Read the model definition and answer for the solid it produces. Units are mm, in the model's axes. A direction names the side the tool comes from. Coordinates: 2 decimals unless noted, no trailing zeros. Loops run counter-clockwise (first coordinate to the right, second up) from the corner with the lowest first, then second, coordinate; pieces in that order, holes last. Notation, with made-up numbers: (8.5, 20.5) -> (38.5, 20.5) arc R17 ccw to (38.5, 51.5) -> close; hole circle Ø2 at (57, 7.25). An arc over 180 degrees is marked (long way). Answer as a JSON object with one key per item and string values. Group by question number.
1) Flat-ended cylindrical pins translate along their axes: P1, Ø4, axis at x = -25.4, y = -63.5, coming from the +Z side; P2, Ø1.4, axis at x = -25, y = -64.5, coming from the -Z side; P3, Ø3, axis at x = 31.75, y = -63.5, coming from the +Z side; P4, Ø5, axis at x = -12.5, y = -17, coming from the +Z side. Find the tip coordinate at first contact, or state that the pin passes through.
2) Which of the six approach directions +Z, -Z, +X, -X, +Y, -Y give full straight-line access (tool end or side, diameter ignored) to faces 4 (the face through (-31.853, -61.153, -6.367)), 5 (the face through (25.297, -65.847, -25.383)), 6 (the face through (-32, -38, 0))?
3) Section C-C, the plane z = -13.5 is taken. Give the vertices of the cut face in (x, y).
4) Consider probe 1 along Y at (x, z) = (-25.4, -28.55); probe 2 along X at (y, z) = (-12.7, -28.05); probe 3 along Y at (x, z) = (31.75, -6.55). Determine where each line is inside the solid, lowest interval first. Write a range as [from, to].
5) Section A-A, the plane z = -1.5 is taken. Give the vertices of the cut face in (x, y), plus the area to 3 significant figures.
6) Section B-B, the plane x = -31.75 is taken. Give the vertices of the cut face in (y, z), plus the area to 3 significant figures.
7) Section D-D, the plane y = -30.5 is taken. Give the vertices of the cut face in (x, z).
8) Determine the mould class of faces 1 (the face through (-23.316, -11.616, -25.383)), 2 (the face through (26.3, -10.53, -25.38)), 3 (the face through (38.1, -38, -16)) for opening direction Y: released by +Y, released by -Y, zero draft, split by the parting line, or undercut.
Autodesk Inventor part; units mm, degrees
ref_plane "YZ Plane" through (0, 0, 0) normal (1, 0, 0) x (0, 1, 0)
ref_plane "XZ Plane" through (0, 0, 0) normal (0, 1, 0) x (-1, 0, 0)
ref_plane "XY Plane" through (0, 0, 0) normal (0, 0, 1) x (1, 0, 0)
sketch "Sketch18" plane through (0, 0, 0) normal (0, 1, 0) x (-1, 0, 0)
  arc A0 (-25.4, 0) -> (25.4, 0) centre (0, 0) ccw
  line L0 (-38.1, 0) -> (-38.1, -31.75)
  line L1 (-38.1, -31.75) -> (38.1, -31.75)
  line L2 (38.1, -31.75) -> (38.1, 0)
  line L3 (38.1, 31.75) -> (-38.1, -31.75) construction
  line L4 (-38.1, 31.75) -> (38.1, -31.75) construction
  line L5 (38.1, 0) -> (25.4, 0)
  line L6 (-25.4, 0) -> (-38.1, 0)
  dimension "d78" = 50.8
  dimension "d79" = 6.35
  dimension "d80" = 12.7
extrude "Extrusion9" add sketch "Sketch18" against normal blind 76.2
sketch "Sketch19" plane through (-38.1, 0, 0) normal (0, 0, 1) x (1, 0, 0)
  line L0 (0, 0) -> (0, -76.2)
  line L1 (12.7, 0) -> (12.7, -76.2)
  line L2 (63.5, 0) -> (63.5, -76.2)
  line L3 (76.2, 0) -> (76.2, -76.2)
  line L4 (76.2, -76.2) -> (63.5, -76.2)
  line L5 (12.7, -76.2) -> (0, -76.2)
  line L6 (0, 0) -> (12.7, 0)
  line L7 (63.5, 0) -> (76.2, 0)
  line L8 (6.35, -63.5) -> (69.85, -63.5) construction
  line L9 (69.85, -63.5) -> (69.85, -12.7) construction
  line L10 (69.85, -12.7) -> (6.35, -12.7) construction
  line L11 (6.35, -12.7) -> (6.35, -63.5) construction
  line L12 (63.5, -76.2) -> (12.7, -76.2) construction
  line L13 (12.7, 0) -> (63.5, 0) construction
  point P0 (38.1, 0)
  dimension "d83" = 6.35
  dimension "d84" = 6.35
  dimension "d85" = 12.7
  dimension "d86" = 12.7
hole "Hole3" at (-31.75, -12.7, 0) at (31.75, -12.7, 0) at (31.75, -63.5, 0) at (-31.75, -63.5, 0) direction (0, 0, -1) diameter 4.699 depth 7.1501 counterbore diameter 4.8514 counterbore depth 5.5626
sketch "Sketch20" plane through (38.1, 0, -31.75) normal (0, 0, -1) x (-1, 0, 0)
  line L0 (76.2, 0) -> (76.2, -76.2)
  line L1 (0, 0) -> (76.2, 0)
  line L2 (0, 0) -> (0, -76.2)
  line L3 (76.2, -76.2) -> (0, -76.2)
  line L4 (12.7, -63.5) -> (63.5, -63.5) construction
  line L5 (63.5, -63.5) -> (63.5, -12.7) construction
  line L6 (63.5, -12.7) -> (12.7, -12.7) construction
  line L7 (12.7, -12.7) -> (12.7, -63.5) construction
  line L8 (12.7, -63.5) -> (63.5, -12.7) construction
  line L9 (63.5, -63.5) -> (12.7, -12.7) construction
  line L10 (0, 0) -> (0, -76.2) construction
  point P0 (38.1, 0)
  point P1 (38.1, -38.1)
  dimension "d94" = 12.7
  dimension "d95" = 12.7
  dimension "d96" = 12.7
  dimension "d97" = 12.7
hole "Hole4" at (25.4, -12.7, -31.75) at (-25.4, -12.7, -31.75) at (-25.4, -63.5, -31.75) at (25.4, -63.5, -31.75) direction (0, 0, 1) diameter 4.699 depth 7.1501 counterbore diameter 4.8514 counterbore depth 5.5626
equation "\"d78\" = legDiameter"
equation "\"d81\" = legPartHeight"
equation "\"legDiameter\" = 50.8"
equation "\"legWalThickness\" = 3.175"
equation "\"legPartHeight\" = 76.2"
properties part number "clampForMeadeTripodLeg"
Determined:
{
 "1": {"P1": "z = 0", "P2": "z = -24.6", "P3": "z = -7.15", "P4": "z = -20.5"},
 "2": {"face 4": "+Z", "face 5": "-Z", "face 6": "+Z, +X, -X, +Y, -Y"},
 "3": {"outline": "(-38.1, -76.2) -> (-21.52, -76.2) -> (-21.52, 0) -> (-38.1, 0) -> close; (21.52, -76.2) -> (38.1, -76.2) -> (38.1, 0) -> (21.52, 0) -> close"},
 "4": {"probe 1": "[-76.2, -65.93], [-61.07, -15.13], [-10.27, 0]", "probe 2": "[-38.1, -27.83], [-22.97, 22.97], [27.83, 38.1]", "probe 3": "[-76.2, -65.85], [-61.15, -15.05], [-10.35, 0]"},
 "5": {"outline": "(-38.1, -76.2) -> (-25.36, -76.2) -> (-25.36, 0) -> (-38.1, 0) -> close; (25.36, -76.2) -> (38.1, -76.2) -> (38.1, 0) -> (25.36, 0) -> close; hole circle Ø4.85 at (-31.75, -63.5); hole circle Ø4.85 at (-31.75, -12.7); hole circle Ø4.85 at (31.75, -63.5); hole circle Ø4.85 at (31.75, -12.7)", "area": "1,870 mm²"},
 "6": {"outline": "(-76.2, -31.75) -> (0, -31.75) -> (0, 0) -> (-10.27, 0) -> (-10.27, -5.56) -> (-10.35, -5.56) -> (-10.35, -7.15) -> (-15.05, -7.15) -> (-15.05, -5.56) -> (-15.13, -5.56) -> (-15.13, 0) -> (-61.07, 0) -> (-61.07, -5.56) -> (-61.15, -5.56) -> (-61.15, -7.15) -> (-65.85, -7.15) -> (-65.85, -5.56) -> (-65.93, -5.56) -> (-65.93, 0) -> (-76.2, 0) -> close", "area": "2,350 mm²"},
 "7": {"outline": "(-38.1, -31.75) -> (38.1, -31.75) -> (38.1, 0) -> (25.4, 0) arc R25.4 cw to (-25.4, 0) -> (-38.1, 0) -> close"},
 "8": {"face 1": "undercut", "face 2": "undercut", "face 3": "zero draft"}
}
